For this review, take the finished solid that the model builds, in its own axes (mm). Face numbers are marked on the shaded views. Give positions to 0.01 mm unless a question says otherwise; leave off trailing zeros. Loops run counter-clockwise (first coordinate to the right, second up) from the corner with the lowest first, then second, coordinate; pieces in that order, holes last. Notation, with made-up numbers: M 47,-33 L 76,-33 A12 cw 76,-20 Z; hole C 4,70.25 d2. An arc over 180 degrees is marked long. Use CSV: the item, a comma, the result in double quotes. Start each with the question number.
1. Take a section at C-C, the plane z = 1.5. Write out the cut boundary in (x, y), and give its area (3 significant figures).
2. Take a section at B-B, the plane y = 100. Write out the cut boundary in (x, z), and give its area (3 significant figures).
3. Take a section at A-A, the plane x = 20. Write out the cut boundary in (y, z).
4. The part is to be moulded in two halves that separate along Y. For the marked faces 1, 2 and 3, say which applies: pulls with the +Y half, pulls with the -Y half, needs draft (parallel to the pull), parting line crosses it, or undercut.
5. Insertion check: P1, Ø2.5, axis at x = 20, y = 100, coming from the +Z side. The pin has a flat end and moves straight along its axis. Give the tip position at first contact, or say it passes through.
6. To check wall thickness, follow line 1 (X direction, y = 100, z = 6.25); line 2 (Y direction, x = 20, z = 7.5); line 3 (Y direction, x = 21, z = 14). State the ranges of each line that lie inside material, in increasing order. Write a range as [from, to].
from build123d import *

# Parameters (mm, degrees)
ESQUISSE1_W                  = 40
ESQUISSE1_H                  = 120
BOSS_EXTRU_1_DEPTH           = 20
CHANFREIN2_SIZE              = 5
ENL_V_MAT_EXTRU_1_DEPTH      = 129.062484749
ENL_V_MAT_EXTRU_1_DEPTH_BACK = 129.062484749
ESQUISSE3_R                  = 2.25


with BuildPart() as part:
    # Esquisse1 → Boss.-Extru.1 (new body)
    with BuildSketch(Plane.XY):
        with Locations((20, 60)):
            Rectangle(ESQUISSE1_W, ESQUISSE1_H)
    extrude(amount=BOSS_EXTRU_1_DEPTH)

    # Chanfrein2
    chanfrein2_edges = [part.edges().sort_by_distance(p)[0] for p in [
        (20, 0, 0),
        (20, 0, 20),
    ]]
    chamfer(chanfrein2_edges, length=CHANFREIN2_SIZE)

    # Esquisse3 → Enlèv. mat.-Extru.1 (cut, two sides: drawn at the far end of the back side and taken through both)
    with BuildSketch(Plane.XY.offset(20).offset(-ENL_V_MAT_EXTRU_1_DEPTH_BACK)):
        with Locations((20, 100)):
            Circle(ESQUISSE3_R)
    extrude(amount=ENL_V_MAT_EXTRU_1_DEPTH + ENL_V_MAT_EXTRU_1_DEPTH_BACK, mode=Mode.SUBTRACT)


solid = part.part
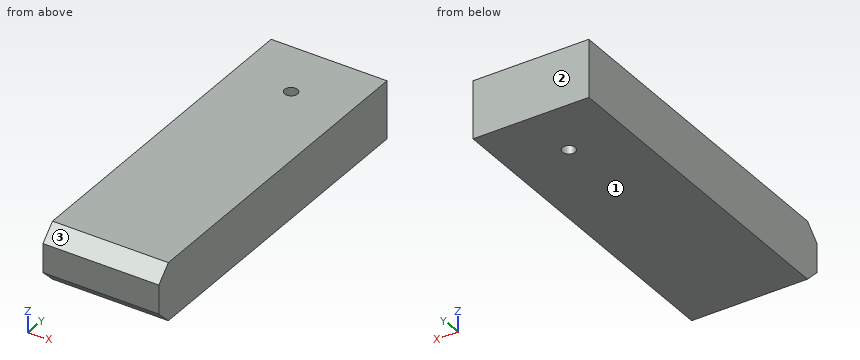
Result set:
1,outline,"M 0,3.5 L 40,3.5 L 40,120 L 0,120 Z; hole C 20,100 d4.5"
1,area,"4,640 mm2"
2,outline,"M 0,0 L 17.75,0 L 17.75,20 L 0,20 Z; M 22.25,0 L 40,0 L 40,20 L 22.25,20 Z"
2,area,"710 mm2"
3,outline,"M 0,5 L 5,0 L 97.75,0 L 97.75,20 L 5,20 L 0,15 Z; M 102.25,0 L 120,0 L 120,20 L 102.25,20 Z"
4,face 1,"needs draft"
4,face 2,"pulls with the +Y half"
4,face 3,"pulls with the -Y half"
5,P1,"through"
6,line 1,"[0, 17.75], [22.25, 40]"
6,line 2,"[0, 97.75], [102.25, 120]"
6,line 3,"[0, 97.98], [102.02, 120]"
